Check sheet for the modelled part. Datum: model origin and axes. Units: mm. Give positions to 0.01 mm unless a question says otherwise; leave off trailing zeros. Order: outer loops, then holes, each group sorted by start corner. A loop starts at its lowest first (then second) coordinate and runs counter-clockwise, first axis right, second up.
Autodesk Inventor part; units mm, degrees
ref_plane "YZ Plane" through (0, 0, 0) normal (1, 0, 0) x (0, 1, 0)
ref_plane "XZ Plane" through (0, 0, 0) normal (0, 1, 0) x (-1, 0, 0)
ref_plane "XY Plane" through (0, 0, 0) normal (0, 0, 1) x (1, 0, 0)
sketch "Sketch1" plane through (0, 0, 0) normal (0, 0, 1) x (1, 0, 0)
  line L0 (21.15, 21.15) -> (21.15, -21.15)
  line L1 (21.15, -21.15) -> (-21.15, -21.15)
  line L2 (-21.15, -21.15) -> (-21.15, 21.15)
  line L3 (-21.15, 21.15) -> (-10, 61.15)
  line L4 (-10, 61.15) -> (10, 61.15)
  line L5 (10, 61.15) -> (21.15, 21.15)
  point P0 (0, 0)
  point P1 (21.15, 0)
  point P2 (0, 61.15)
  dimension "d0" = 42.3
  dimension "d1" = 42.3
  dimension "d2" = 20
  dimension "d4" = 42.3
  dimension "d5" = 40
  dimension "d7" = 11.15
extrude "Extrusion1" add sketch "Sketch1" along normal blind 4
sketch "Sketch2" plane through (0, 0, 4) normal (0, 0, 1) x (1, 0, 0)
  line L0 (10, 61.15) -> (-10, 61.15)
  point P0 (0, 0)
  point P1 (0, 51.15)
  point P2 (0, 36.15)
  dimension "d10" = 10
  dimension "d11" = 15
hole "Hole1" at (0, 51.15, 4) at (0, 36.15, 4) direction (0, 0, -1) diameter 4.5 end through all
sketch "Sketch3" plane through (0, 0, 4) normal (0, 0, 1) x (1, 0, 0)
  circle A0 centre (0, 0) radius 12
  dimension "d19" = 24
extrude "Extrusion2" cut sketch "Sketch3" against normal through all
sketch "Sketch4" plane through (0, 0, 4) normal (0, 0, 1) x (1, 0, 0)
  line L0 (-21.15, 21.15) -> (-21.15, -21.15)
  line L1 (-21.15, -21.15) -> (21.15, -21.15)
  point P0 (0, 0)
  point P1 (-15.5, 15.5)
  point P2 (15.5, 15.5)
  point P3 (15.5, -15.5)
  point P4 (-15.5, -15.5)
  dimension "d22" = 31
  dimension "d23" = 31
  dimension "d24" = 5.65
  dimension "d25" = 5.65
hole "Hole2" at (-15.5, 15.5, 4) at (15.5, 15.5, 4) at (15.5, -15.5, 4) at (-15.5, -15.5, 4) direction (0, 0, -1) diameter 3 end through all
properties part number "Stepper Motor to Extrusion Clip"
(1) Cross-section at C-C on z = 3.15. Enter the section's corners in (x, y).
Response values:
outline: (-21.15, -21.15) - (21.15, -21.15) - (21.15, 21.15) - (10, 61.15) - (-10, 61.15) - (-21.15, 21.15) - close; hole circle Ø3 at (-15.5, -15.5); hole circle Ø3 at (-15.5, 15.5); hole circle Ø24 at (0, 0); hole circle Ø4.5 at (0, 36.15); hole circle Ø4.5 at (0, 51.15); hole circle Ø3 at (15.5, -15.5); hole circle Ø3 at (15.5, 15.5)
(2) Cross-section at D-D on y = 11. Enter the section's corners in (x, z).
Response values:
outline: (-21.15, 0) - (-4.8, 0) - (-4.8, 4) - (-21.15, 4) - close; (4.8, 0) - (21.15, 0) - (21.15, 4) - (4.8, 4) - close
(3) Cross-section at B-B on x = -8.5. Enter the section's corners in (y, z).
Response values:
outline: (-21.15, 0) - (-8.47, 0) - (-8.47, 4) - (-21.15, 4) - close; (8.47, 0) - (61.15, 0) - (61.15, 4) - (8.47, 4) - close
(4) Material ranges on L1, parallel to X at y = 15.5, z = 1.95; L2, parallel to Y at x = 0, z = 1.95; L3, parallel to Y at x = 1, z = 2.3, recorded low to high.
Response values:
L1: x = -21.15 to -17, -14 to 14, 17 to 21.15
L2: y = -21.15 to -12, 12 to 33.9, 38.4 to 48.9, 53.4 to 61.15
L3: y = -21.15 to -11.96, 11.96 to 34.13, 38.17 to 49.13, 53.17 to 61.15
(5) Release check for a two-part mould opening along Y. For faces 1 (the face through (-0.676, 49.004, 1.972)), 2 (the face through (-21.15, 0, 2)), 3 (the face through (15.43, -14, 1.97)), 4 (the face through (15.497, 41.43, 1.972)) record: released by +Y, released by -Y, zero draft, split by the parting line, or undercut.
Response values:
face 1: undercut
face 2: zero draft
face 3: undercut
face 4: released by +Y
(6) Cross-section at A-A on y = -15.5. Enter the section's corners in (x, z), then the cut area to 3 significant figures.
Response values:
outline: (-21.15, 0) - (-17, 0) - (-17, 4) - (-21.15, 4) - close; (-14, 0) - (14, 0) - (14, 4) - (-14, 4) - close; (17, 0) - (21.15, 0) - (21.15, 4) - (17, 4) - close
area: 145 mm2
